```python
from build123d import *

# Parameters (mm, degrees)
SKETCH1_R           = 94.2975
SKETCH1_R_2         = 89.662
BOSS_EXTRUDE1_DEPTH = 203.2
SKETCH5_W           = 3.429
SKETCH5_H           = 5.08
SKETCH5_W_2         = 5.08
SKETCH5_H_2         = 3.429
CUT_EXTRUDE1_DEPTH  = 203.2
CUT_EXTRUDE2_START  = -12.7
CUT_EXTRUDE2_DEPTH  = 184.15
CIRPATTERN1_COUNT   = 4
FILLET1_R           = 2.54


with BuildPart() as part:
    # Sketch1 → Boss-Extrude1 (new body)
    with BuildSketch(Plane(origin=(0, 0, 0), x_dir=(1, 0, 0), z_dir=(0, 1, 0))):
        Circle(SKETCH1_R)
        Circle(SKETCH1_R_2, mode=Mode.SUBTRACT)
    extrude(amount=-BOSS_EXTRUDE1_DEPTH)

    # Sketch5 → Cut-Extrude1 (cut)
    with BuildSketch(Plane(origin=(0, 0, 0), x_dir=(1, 0, 0), z_dir=(0, 1, 0))):
        with Locations((0, 93.360875)):
            Rectangle(SKETCH5_W, SKETCH5_H)
        with Locations((0, -93.360875)):
            Rectangle(SKETCH5_W, SKETCH5_H)
        with Locations((-93.360875, -0.0635)):
            Rectangle(SKETCH5_W_2, SKETCH5_H_2)
        with Locations((93.360875, -0.0635)):
            Rectangle(SKETCH5_W_2, SKETCH5_H_2)
    extrude(amount=-CUT_EXTRUDE1_DEPTH, mode=Mode.SUBTRACT)

    # Sketch7 → Cut-Extrude2 (cut)
    with BuildSketch(Plane(origin=(0, 0, 0), x_dir=(1, 0, 0), z_dir=(0, 1, 0)).offset(CUT_EXTRUDE2_START)):
        with BuildLine():
            Line((89.292832075, -8.128), (93.946549283, -8.128))
            ThreePointArc((93.946549283, -8.128), (66.655864041, -66.700931742), (8.0645, -93.952021511))
            Line((8.0645, -93.952021511), (8.0645, -89.298589484))
            ThreePointArc((8.0645, -89.298589484), (63.378061476, -63.423146938), (89.292832075, -8.128))
        make_face()
    cut_extrude2 = extrude(amount=-CUT_EXTRUDE2_DEPTH, mode=Mode.SUBTRACT)

    # CirPattern1: Cut-Extrude2 ×4 about axis
    cirpattern1_axis = Axis((0, 0, 0), (0, 1, 0))
    for i in range(1, CIRPATTERN1_COUNT):
        add(cut_extrude2.rotate(cirpattern1_axis, i * 360 / CIRPATTERN1_COUNT), mode=Mode.SUBTRACT)

    # Fillet1
    fillet1_edges = [part.edges().sort_by_distance(p)[0] for p in [
        (66.700852134, 0, -66.655943702),
        (-66.700852134, 0, -66.655943702),
        (-66.655943427, 0, 66.700852409),
        (66.655943427, 0, 66.700852409),
    ]]
    fillet(fillet1_edges, radius=FILLET1_R)


solid = part.part
```
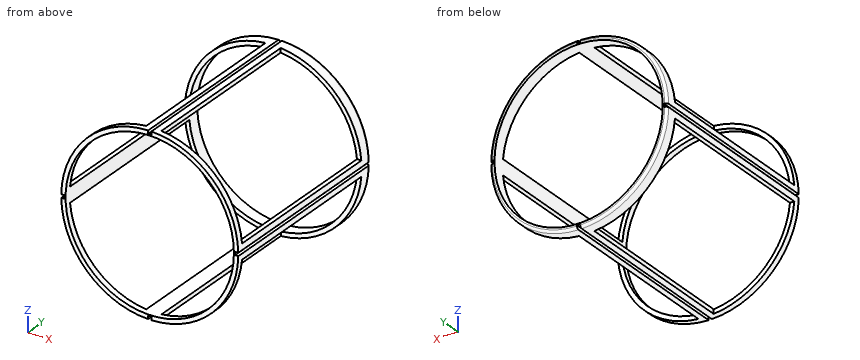
Check sheet for the modelled part. Datum: model origin and axes. Units: mm. Round coordinates to 2 decimals unless told otherwise and drop trailing zeros. Answer as CSV lines item,"result". Start each with the question number.
1) Depth check by flat-ended pin: pin 1 (1 mm diameter, centred on y = -91.5, z = 0.5, fed in from -X); pin 2 (2.5 mm diameter, centred on x = -92, y = -134, fed in from -Z); pin 3 (1.7 mm diameter, centred on x = 0, y = -127, fed in from +Z); pin 4 (2 mm diameter, centred on x = -63.5, z = 70, fed in from -Y). Enter the tip coordinate at first touch or a pass-through.
2) Scan lines: probe 1 along X at (y, z) = (-136, 0); probe 2 along Y at (x, z) = (83.5, 37). Record each from-to range of solid material in increasing order.
3) Section check A-A (y = -41.5). Give the number of separate pieces and of enclosed holes in the cut face, then the cut area to 3 significant figures.
Determined:
1,pin 1,"x = -90.82"
1,pin 2,"z = -8.13"
1,pin 3,"z = 90.82"
1,pin 4,"y = -203.2"
2,probe 1,"-90.82 to -89.66, 89.66 to 90.82"
2,probe 2,"-203.2 to -196.85, -12.7 to 0"
3,separate pieces,"4"
3,enclosed holes,"0"
3,area,"253 mm^2"
